```python
from build123d import *

# Parameters (mm, degrees)
F1_DEPTH    = 25
F2_R        = 10
F3_T1_DEPTH = 25
F4_R        = 2
F5_W        = 19
F5_H        = 10
F5_W_2      = 13
F5_H_2      = 4
F6_DEPTH    = 2


# Not quite as in the source:
# - a fillet or chamfer that OpenCascade refuses, or shapes differently, is made with other operations: its cross-section is extruded or revolved along the edge and cut away or added


with BuildPart() as f1:
    # F0 (on Right) → F1 (new body)
    with BuildSketch(Plane.YZ):
        with BuildLine():
            Line((-119.9998666872, 30.0034820876), (-120, 0))
            Line((-120, 0), (0, 0))
            Line((0, 0), (0, 90))
            Line((0, 90), (-120, 90))
            Line((-120, 90), (-120, 70))
            Line((-120, 70), (-20, 70))
            Line((-20, 70), (-20, 20.003633132))
            ThreePointArc((-20, 20.003633132), (-24.9999333448, 15.0036997872), (-29.9998666895, 20.003633132))
            Line((-29.9998666895, 20.003633132), (-34.9998666895, 20.003633132))
            ThreePointArc((-34.9998666895, 20.003633132), (-39.9998666895, 15.003633132), (-44.9998666895, 20.003633132))
            Line((-44.9998666895, 20.003633132), (-49.9998666872, 20.0034820876))
            ThreePointArc((-49.9998666872, 20.0034820876), (-54.9998666872, 15.0034820876), (-59.9998666872, 20.0034820876))
            Line((-59.9998666872, 20.0034820876), (-64.9998666872, 20.0034820876))
            ThreePointArc((-64.9998666872, 20.0034820876), (-69.9998666872, 15.0034820876), (-74.9998666872, 20.0034820876))
            Line((-74.9998666872, 20.0034820876), (-79.9998666872, 20.0034820876))
            ThreePointArc((-79.9998666872, 20.0034820876), (-84.9998666872, 15.0034820876), (-89.9998666872, 20.0034820876))
            Line((-89.9998666872, 20.0034820876), (-94.9998666872, 20.0034820876))
            ThreePointArc((-94.9998666872, 20.0034820876), (-99.9998666872, 15.0034820876), (-104.9998666872, 20.0034820876))
            Line((-104.9998666872, 20.0034820876), (-109.9998666872, 20.0034820876))
            Line((-109.9998666872, 20.0034820876), (-109.9998666872, 30.0034820876))
            Line((-109.9998666872, 30.0034820876), (-119.9998666872, 30.0034820876))
        make_face()
    extrude(amount=F1_DEPTH)

    # F2
    f2_edges = [f1.edges().sort_by_distance(p)[0] for p in [
        (12.5, -120, 90),
        (12.5, 0, 90),
        (12.5, 0, 0),
        (12.5, -120, 0),
    ]]
    fillet(f2_edges, radius=F2_R)

    # F3: fillet of radius 10 on 1 edges, made by hand

    # F3_s2 → F3_t1 (join)
    with BuildSketch(Plane.YZ):
        with BuildLine():
            add(Edge.make_bspline(
                [(-30, 70), (-20, 70), (-20, 60)],
                knots=[0, 0, 0, 1, 1, 1], degree=2, weights=[1, 1, 1]))
            Line((-20, 60), (-20, 70))
            Line((-20, 70), (-30, 70))
        make_face()
    extrude(amount=F3_T1_DEPTH)

    # F4
    f4_edges = [f1.edges().sort_by_distance(p)[0] for p in [
        (12.5, -119.999867, 30.003482),
        (12.5, -109.999867, 30.003482),
        (12.5, -109.999867, 20.003482),
        (12.5, -104.999867, 20.003482),
        (12.5, -94.999867, 20.003482),
        (12.5, -89.999867, 20.003482),
        (12.5, -79.999867, 20.003482),
        (12.5, -74.999867, 20.003482),
        (12.5, -64.999867, 20.003482),
        (12.5, -59.999867, 20.003482),
        (12.5, -49.999867, 20.003482),
        (12.5, -44.999867, 20.003633),
        (12.5, -34.999867, 20.003633),
        (12.5, -29.999867, 20.003633),
    ]]
    fillet(f4_edges, radius=F4_R)

    # F5 (on face) → F6 (join)
    with BuildSketch(Plane(origin=(0, 0, 0), x_dir=(-1, 0, 0), z_dir=(0, 1, 0))):
        Polygon((-22, 16), (-22, 13), (-3, 13), (-3, 16), (-11, 16), (-11, 21), (-3, 21), (-3, 24), (-22, 24), (-22, 21), (-14, 21), (-14, 16), align=None)
        with Locations((-12.5, 32)):
            Rectangle(F5_W, F5_H)
        with Locations((-12.5, 32)):
            Rectangle(F5_W_2, F5_H_2, mode=Mode.SUBTRACT)
        with Locations((-12.5, 45)):
            Rectangle(F5_W, F5_H)
        with Locations((-12.5, 45)):
            Rectangle(F5_W_2, F5_H_2, mode=Mode.SUBTRACT)
        Polygon((-22, 56), (-22, 53), (-3, 53), (-3, 56), (-10.7311028987, 56), (-3, 61), (-3, 64), (-12.5, 59), (-22, 64), (-22, 61), (-12.5, 56), align=None)
        Polygon((-22, 72), (-3, 65.6102970243), (-3, 68.6102970243), (-8.8134625163, 70.7304688778), (-8.5728853775, 72.4904765496), (-3, 74), (-3, 77), align=None)
    extrude(amount=F6_DEPTH)


solid = f1.part
```
Here's how the part is built. I have some questions about the finished solid (model axes, mm). A direction names the side the tool comes from. Give positions to 0.01 mm unless a question says otherwise; leave off trailing zeros. Loops run counter-clockwise (first coordinate to the right, second up) from the corner with the lowest first, then second, coordinate; pieces in that order, holes last. Notation, with made-up numbers: M 52,0 L 101,0 A12 cw 101,4 Z; hole C 33.25,7.25 d3. An arc over 180 degrees is marked long. Use one line per item in the form item = value. Start each with the question number.
Q1. If we section it at D-D (z = 83.5): Write out the boundary of the cut face in (x, y), then the cut area to 3 significant figures.
Q2. If we section it at C-C (y = -72.5): Write out the boundary of the cut face in (x, z), then the cut area to 3 significant figures.
Q3. I need wall thicknesses on line 1 along Z through (x, y) = (3.5, -58); line 2 along Z through (x, y) = (7.5, -99.5); line 3 along Y through (x, z) = (14, 58.5). Which ranges of each line are inside material? Lowest first, please.
Q4. If we section it at A-A (z = 48.5): Write out the boundary of the cut face in (x, y).
Q5. If we section it at B-B (y = -86.5): Write out the boundary of the cut face in (x, z).
Q6. Will these pins go through, and if not, where does the flat tip stop? pin 1 Ø0.6 at (x, y) = (10, 1.5) entering from +Z; pin 2 Ø1.6 at (x, y) = (10, 1) entering from -Z; pin 3 Ø2 at (x, z) = (13.5, 32.5) entering from +Y.
Q7. Thinking about a two-plate mould opening in Z: for faces 5 (the flat face through (17.316, 0.986, 58.535)), 6 (the cylindrical face through (12.68, -2.85, 86.99)), 7 (the cylindrical face through (12.325, -84.91, 15.004)), 8 (the flat face through (12, -120, 75)), which applies, +Z half, -Z half, draft (parallel to the pull), parting line (faces both ways), or undercut?
Q8. Which directions (+Z, -Z, +X, -X, +Y, -Y) give clear straight access to the entire face, cutting with the end or side of a thin tool? Please do faces 1 (the cylindrical face through (12.325, -54.91, 15.004)), 2 (the flat face through (12, -76, 70)), 3 (the flat face through (12.367, 0.986, 74.535)), 4 (the flat face through (17.184, 0.986, 61.465)).
Taken from the geometry:
q1.outline = M 0,-119.37 L 25,-119.37 L 25,-0.63 L 0,-0.63 Z
q1.area = 2,970 mm^2
q2.outline = M 0,0 L 25,0 L 25,15.67 L 0,15.67 Z; M 0,70 L 25,70 L 25,90 L 0,90 Z
q2.area = 892 mm^2
q3.line_1 = 0 to 16, 70 to 90
q3.line_2 = 0 to 15.03, 70 to 90
q3.line_3 = -20 to 2
q4.outline = M 0,-20 L 25,-20 L 25,0 L 22,0 L 22,2 L 3,2 L 3,0 L 0,0 Z
q5.outline = M 0,0 L 25,0 L 25,15.23 L 0,15.23 Z; M 0,70 L 25,70 L 25,90 L 0,90 Z
q6.pin_1 = 75.24
q6.pin_2 = 13
q6.pin_3 = 0
q7.face_5 = undercut
q7.face_6 = +Z half
q7.face_7 = undercut
q7.face_8 = draft
q8.face_1 = +X, -X
q8.face_2 = +X, -X, -Y
q8.face_3 = +Z, +X, +Y
q8.face_4 = +Y
